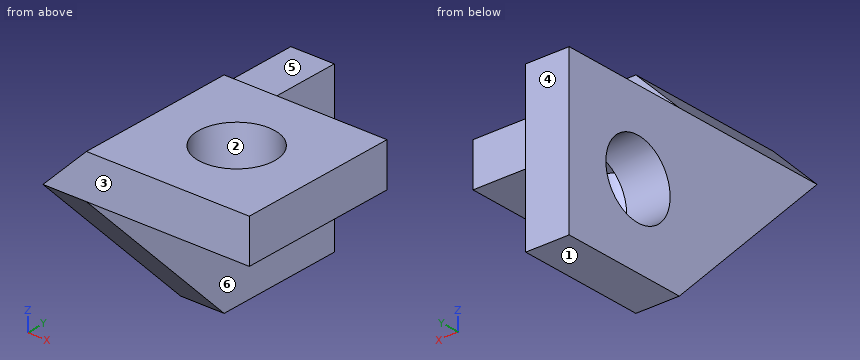
Autodesk Inventor part; units mm, degrees
ref_plane "YZ Plane" through (0, 0, 0) normal (1, 0, 0) x (0, 1, 0)
ref_plane "XZ Plane" through (0, 0, 0) normal (0, 1, 0) x (-1, 0, 0)
ref_plane "XY Plane" through (0, 0, 0) normal (0, 0, 1) x (1, 0, 0)
sketch "Boceto2" plane through (0, 0, 0) normal (0, 0, 1) x (1, 0, 0)
  line L0 (0, 0) -> (2, 0)
  line L1 (2, 0) -> (2, -7.5)
  line L2 (2, 0) -> (3, 0)
  line L3 (2.8119, -7.5) -> (0, -7.5)
  line L4 (0, -7.5) -> (0, 0)
  line L5 (3, 0) -> (3, -7.5)
  line L6 (3, -7.5) -> (0, -7.5)
  line L7 (3, 0) -> (6.5, 0)
  line L8 (6.5, 0) -> (8.5, 0)
  line L9 (8.5, 0) -> (8.5, -7.5)
  line L10 (8.5, -7.5) -> (3, -7.5)
  circle A0 centre (5.75, -3.75) radius 1.75
  dimension "d6" = 2
  dimension "d15" = 1
  dimension "d16" = 3.5
  dimension "d17" = 2
  dimension "d18" = 3.5
sketch "Boceto1" plane through (0, 0, 0) normal (1, 0, 0) x (0, 1, 0)
  line L0 (0, 0) -> (0, -2)
  line L1 (0, -2) -> (0, -5.5)
  line L2 (0, -5.5) -> (0, -7.5)
  line L3 (0, -7.5) -> (-2, -7.5)
  line L4 (-2, -7.5) -> (-5.5, -7.5)
  line L5 (0, 0) -> (-5.5, 0)
  line L6 (-5.5, -7.5) -> (-7.5, -7.5)
  line L7 (-7.5, -7.5) -> (-7.5, 0)
  line L8 (-7.5, 0) -> (0, 0)
  dimension "d0" = 2
  dimension "d1" = 3.5
  dimension "d2" = 2
  dimension "d3" = 2
  dimension "d4" = 3.5
  dimension "d5" = 2
extrude "Extrusión2" add sketch "Boceto2" along normal blind 2
chamfer "Chaflán1" distance 2 angle 45 1 edges at (0, -3.75, 2)
sketch "Boceto4" plane through (0, 0, 2) normal (0, 0, 1) x (1, 0, 0)
  line L0 (8.5, -7.5) -> (9.5, -7.5)
  line L1 (9.5, -7.5) -> (9.5, 0)
  line L2 (9.5, 0) -> (8.5, 0)
  line L3 (8.5, -7.5) -> (8.5, 0)
  line L4 (8.5, 0) -> (8.5, -7.5)
  point P0 (0, 0)
  dimension "d24" = 1
extrude "Extrusión3" add sketch "Boceto4" against normal blind 2
ref_plane "Plano de trabajo2" through (0, 0, -7.5) normal (0, 1, 0) x (1, 0, 0)
sketch "Boceto5" plane through (0, 0, -7.5) normal (0, 1, 0) x (1, 0, 0)
  line L0 (0, -7.5) -> (2, -9.5)
  line L1 (0, -7.5) -> (2, -7.5)
  line L2 (2, -7.5) -> (2, 0)
  line L3 (2, -7.5) -> (2, 0)
  line L4 (0, 0) -> (2, 0)
  line L5 (2, 0) -> (0, 0)
  line L6 (2, -7.5) -> (2, -9.5)
  line L7 (0, 0) -> (0, -7.5)
  line L8 (0, -7.5) -> (0, 0)
extrude "Extrusión4" add sketch "Boceto5" along normal blind 6
extrude "Extrusión5" cut sketch "Boceto1" along normal blind 2
extrude "Extrusión6" add sketch "Boceto1" along normal blind 2
sketch "Boceto6" plane through (0, -7.5, -7.5) normal (-1, 0, 0) x (0, 0, 1)
  line L0 (0, 13.5) -> (7.5, 13.5)
  line L1 (3.75, 13.5) -> (3.75, 11.5)
  line L2 (3.75, 11.5) -> (3.75, 8)
  circle A0 centre (3.75, 9.75) radius 1.75
  point P0 (7.5, 7.5)
  dimension "d33" = 3.5
extrude "Extrusión7" cut sketch "Boceto6" against normal blind 29.5
sketch "Boceto7" plane through (0, 6, -7.5) normal (0, 1, 0) x (1, 0, 0)
  line L0 (0, 0) -> (0, -7.5)
  line L1 (0, -7.5) -> (2, -7.5)
  line L2 (2, -9.5) -> (2, 0)
  line L3 (2, -7.5) -> (2, -9.5)
  line L4 (0, -7.5) -> (2, -9.5)
  line L5 (2, -9.5) -> (0, -7.5)
extrude "Extrusión8" cut sketch "Boceto7" against normal blind 6
chamfer "Chaflán2" distance 7.5 angle 45 1 edges at (1, -7.5, -7.5)
properties part number "Caixa control - tirador"
For this review, take the finished solid that the model builds, in its own axes (mm). Face numbers are marked on the shaded views. A direction names the side the tool comes from. Give positions to 0.01 mm unless a question says otherwise; leave off trailing zeros. Loops run counter-clockwise (first coordinate to the right, second up) from the corner with the lowest first, then second, coordinate; pieces in that order, holes last. Notation, with made-up numbers: (30.5, 83.25) -> (83.5, 83.25) arc R29 ccw to (83.5, 108.25) -> close; hole circle Ø8 at (-11.5, 28.25). An arc over 180 degrees is marked (long way). One line per question, with ' | ' between items.
1) To check wall thickness, follow probe 1 along Y at (x, z) = (5.75, 0.8); probe 2 along Z at (x, y) = (5, -5.5). State the ranges of each line that lie inside material, in increasing order.
Resolved:
probe 1: y = -7.5 to -5.5, -2 to 0 | probe 2: z = 0 to 2
2) We need section D-D (x = 1). Write out the cut boundary in (y, z).
Resolved:
outline: (-7.5, 0) -> (0, -7.5) -> (6, -7.5) -> (6, 0) -> (0, 0) -> (0, 1) -> (-7.5, 1) -> close; hole circle Ø3.5 at (2.25, -3.75)
3) We need section A-A (y = -3.75). Write out the cut boundary in (x, z).
Resolved:
outline: (0, -3.75) -> (2, -3.75) -> (2, 0) -> (4, 0) -> (4, 2) -> (2, 2) -> (0, 0) -> close; (7.5, 0) -> (9.5, 0) -> (9.5, 2) -> (7.5, 2) -> close
4) The part is to be moulded in two halves that separate along Y. For the marked faces 1, 2 and 3, say which applies: +Y half, -Y half, draft (parallel to the pull), parting line (faces both ways), or undercut.
Resolved:
face 1: draft | face 2: undercut | face 3: -Y half
5) For the marked faces 4, 5 and 6, list the 3-axis set-ups (+Z, -Z, +X, -X, +Y, -Y) from which the entire face can be reached by the end or side of a thin tool; tool diameter is ignored.
Resolved:
face 4: +Z, -Z, +X, -X, +Y | face 5: +Z, +X, -X, +Y | face 6: -Z, +X, +Y, -Y
6) We need section C-C (x = 5.75). Write out the cut boundary in (y, z), plus the area to 3 significant figures.
Resolved:
outline: (-7.5, 0) -> (-5.5, 0) -> (-5.5, 2) -> (-7.5, 2) -> close; (-2, 0) -> (0, 0) -> (0, 2) -> (-2, 2) -> close | area: 8.00 mm2
7) Insertion check: pin 1 Ø4.5 at (x, y) = (5.75, -3.75) entering from +Z; pin 2 Ø4 at (y, z) = (2, -2.5) entering from +X; pin 3 Ø1 at (x, y) = (1.5, 2) entering from +Z; pin 4 Ø1 at (x, z) = (5.5, 1.5) entering from +Y. Each pin has a flat end and moves straight along its axis. Give the tip position at first contact, or say it passes through.
Resolved:
pin 1: stops at z = 2 | pin 2: stops at x = 2 | pin 3: stops at z = 0 | pin 4: stops at y = 0
8) We need section B-B (z = -3.75). Write out the cut boundary in (x, y).
Resolved:
outline: (0, -3.75) -> (2, -3.75) -> (2, 0.5) -> (0, 0.5) -> close; (0, 4) -> (2, 4) -> (2, 6) -> (0, 6) -> close
